Check sheet for the modelled part. Datum: model origin and axes. Units: mm. Face numbers are marked on the shaded views. A direction names the side the tool comes from. Round coordinates to 2 decimals unless told otherwise and drop trailing zeros. Order: outer loops, then holes, each group sorted by start corner. A loop starts at its lowest first (then second) coordinate and runs counter-clockwise, first axis right, second up. Notation, with made-up numbers: (82.25, -15) -> (138.25, -15) arc R28 ccw to (138.25, 17) -> close; hole circle Ø3 at (4.5, -40). An arc over 180 degrees is marked (long way). Answer in a Markdown table with one row per item.
from build123d import *

# Parameters (mm, degrees)
SKETCH1_R           = 6
BOSS_EXTRUDE1_DEPTH = 27
BOSS_EXTRUDE2_START = 11
BOSS_EXTRUDE2_DEPTH = 11
SKETCH3_R           = 1.75
CUT_EXTRUDE1_DEPTH  = 6
SKETCH4_R           = 7.5
BOSS_EXTRUDE3_DEPTH = 15
CHAMFER1_SIZE2      = 1.5
CHAMFER1_SIZE       = 4.121216129


with BuildPart() as part:
    # Sketch1 → Boss-Extrude1 (new body)
    with BuildSketch(Plane.XY):
        Circle(SKETCH1_R)
    extrude(amount=BOSS_EXTRUDE1_DEPTH)

    # Sketch2 → Boss-Extrude2 (add)
    with BuildSketch(Plane(origin=(0, 0, 0), x_dir=(-1, 0, 0), z_dir=(0, 0, -1)).offset(BOSS_EXTRUDE2_START)):
        with BuildLine():
            Line((-1.25, -5.868347297), (-1.25, 5.868347297))
            ThreePointArc((-1.25, 5.868347297), (0, 6), (1.25, 5.868347297))
            Line((1.25, 5.868347297), (1.25, -5.868347297))
            ThreePointArc((1.25, -5.868347297), (0, -6), (-1.25, -5.868347297))
        make_face()
    extrude(amount=-BOSS_EXTRUDE2_DEPTH)

    # Sketch3 → Cut-Extrude1 (cut)
    with BuildSketch(Plane(origin=(1.25, 0, 0), x_dir=(0, 0, -1), z_dir=(1, 0, 0))):
        with Locations((3, 0)):
            Circle(SKETCH3_R)
    extrude(amount=-CUT_EXTRUDE1_DEPTH, mode=Mode.SUBTRACT)

    # Sketch4 → Boss-Extrude3 (add)
    with BuildSketch(Plane.XY.offset(27)):
        Circle(SKETCH4_R)
    extrude(amount=BOSS_EXTRUDE3_DEPTH)

    # Chamfer1
    chamfer1_edges = [part.edges().sort_by_distance(p)[0] for p in [
        (-7.5, 0, 27),
    ]]
    chamfer1_side = [part.faces().sort_by_distance(p)[0] for p in [
        (-7.5, 0, 27.03),
    ]]
    chamfer(chamfer1_edges, length=CHAMFER1_SIZE - 0.0001, length2=CHAMFER1_SIZE2 - 0.0001, reference=chamfer1_side[0])  # a hair under: the kernel refuses the full size


solid = part.part
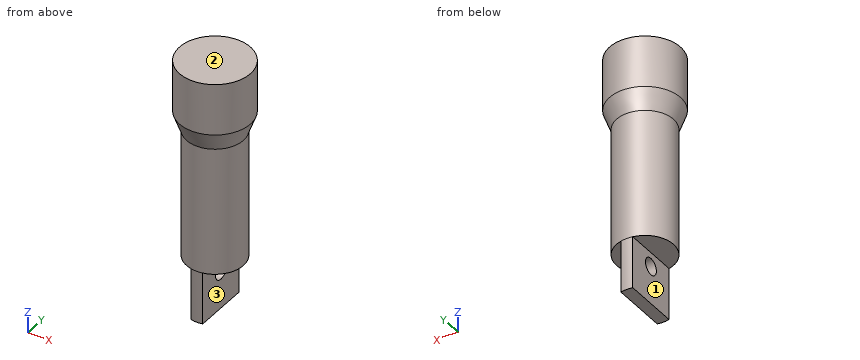
Item 1: Cross-section at D-D (z = 32). Record the boundary of the cut face in (x, y), and give its area (3 significant figures).
Result sheet:
| item | result |
|---|---|
| outline | circle Ø15 at (0, 0) |
| area | 177 mm^2 |
Item 2: Set-up check for the marked faces 1, 2 and 3: record each of +Z, -Z, +X, -X, +Y, -Y from which the full face is reachable in a straight line by a thin tool's end or side.
Result sheet:
| item | result |
|---|---|
| face 1 | -Z, -X, +Y, -Y |
| face 2 | +Z, +X, -X, +Y, -Y |
| face 3 | -Z, +X, +Y, -Y |
Item 3: Cross-section at B-B (z = -3). Record the boundary of the cut face in (x, y).
Result sheet:
| item | result |
|---|---|
| outline | (-1.25, -5.87) arc R6 ccw to (1.25, -5.87) -> (1.25, -1.75) -> (-1.25, -1.75) -> close; (-1.25, 1.75) -> (1.25, 1.75) -> (1.25, 5.87) arc R6 ccw to (-1.25, 5.87) -> close |
Item 4: Scan lines: line 1 (Y direction, x = 0.3, z = -3); line 2 (X direction, y = 5.25, z = -7.5); line 3 (Z direction, x = 5.25, y = -1). Record each from-to range of solid material in increasing order. Write a range as [from, to].
Result sheet:
| item | result |
|---|---|
| line 1 | y = [-5.99, -1.75], [1.75, 5.99] |
| line 2 | x = [-1.25, 1.25] |
| line 3 | z = [0, 42] |
Item 5: Depth check by flat-ended pin: P1, Ø2, axis at y = -6, z = 14.5, coming from the +X side; P2, Ø9, axis at y = -2.5, z = -3.5, coming from the +X side; P3, Ø2, axis at y = -4.5, z = 35, coming from the +X side. Enter the tip coordinate at first touch or a pass-through.
Result sheet:
| item | result |
|---|---|
| P1 | stops at x = 3.32 |
| P2 | stops at x = 6 |
| P3 | stops at x = 6.63 |
